Autodesk Inventor part; units mm, degrees
ref_plane "YZ Plane" through (0, 0, 0) normal (1, 0, 0) x (0, 1, 0)
ref_plane "XZ Plane" through (0, 0, 0) normal (0, 1, 0) x (-1, 0, 0)
ref_plane "XY Plane" through (0, 0, 0) normal (0, 0, 1) x (1, 0, 0)
sketch "スケッチ1" plane through (0, 0, 0) normal (0, 1, 0) x (-1, 0, 0)
  line L0 (-6, -5) -> (6, -5)
  line L1 (6, -5) -> (6, 5)
  line L2 (6, 5) -> (-6, 5)
  line L3 (-6, 5) -> (-6, -5)
  line L4 (-6, -5) -> (6, 5) construction
  line L5 (6, -5) -> (-6, 5) construction
  point P0 (0, 0)
  dimension "d0" = 12
  dimension "d1" = 10
extrude "押し出し1" add sketch "スケッチ1" along normal blind 10
sketch "スケッチ3" plane through (0, 10, 0) normal (0, 1, 0) x (1, 0, 0)
  line L0 (6, -5) -> (6, 5)
  line L1 (-6, 5) -> (-6, -5)
  point P0 (0, 0)
  point P1 (3, 0)
  point P2 (-3, 0)
  point P3 (-6, 0)
  dimension "d4" = 3
  dimension "d12" = 3
hole "穴1" at (3, 10, 0) at (-3, 10, 0) direction (0, -1, 0) diameter 3 end through all
sketch "スケッチ4" plane through (6, 0, -5) normal (0, 0, -1) x (-1, 0, 0)
  line L0 (0, 0) -> (12, 0)
  line L1 (12, 0) -> (12, 10)
  point P0 (6, 0)
  point P1 (6, 5)
  point P2 (6, 0)
  point P3 (12, 5)
hole "穴2" at (0, 5, -5) direction (0, 0, 1) diameter 3 end through all
sketch "スケッチ5" plane through (6, 0, 5) normal (1, 0, 0) x (0, 0, -1)
  line L0 (1, 1) -> (9, 1)
  line L1 (9, 1) -> (9, 9)
  line L2 (9, 9) -> (1, 9)
  line L3 (1, 9) -> (1, 1)
  line L4 (1, 1) -> (9, 9) construction
  line L5 (9, 1) -> (1, 9) construction
  line L6 (10, 0) -> (10, 10)
  point P0 (5, 0)
  point P1 (5, 5)
  point P2 (5, 5)
  point P3 (5, 5)
  point P4 (10, 5)
  dimension "d20" = 8
  dimension "d21" = 8
extrude "押し出し2" cut sketch "スケッチ5" against normal blind 12
properties part number "sensor_attach" material "アルミニウム 6061"
Design review of the part built by this model. Coordinates are the model's own, in mm. A direction names the side the tool comes from. Give positions to 0.01 mm unless a question says otherwise; leave off trailing zeros. Order: outer loops, then holes, each group sorted by start corner. A loop starts at its lowest first (then second) coordinate and runs counter-clockwise, first axis right, second up. Notation, with made-up numbers: (-20.75, 88) -> (30.25, 88) arc R16 cw to (30.25, 113) -> close; hole circle Ø6 at (-7.75, 87.25). An arc over 180 degrees is marked (long way). Write each question's results on one line, items separated by ' | '. Start each with the question number.
Q1. Add section A-A on z = -2. Give the boundary of the cut face in (x, y).
Q2. Wall thickness on L1, parallel to Z at x = -3, y = 0.35; L2, parallel to Y at x = -1.75, z = 3; L3, parallel to Z at x = -4.25, y = 2: over which ranges is each line inside the solid? List them lowest first. Write a range as from..to.
Q3. For pin 1 (2.5 mm diameter, centred on x = -3, z = 0, fed in from -Y); pin 2 (5 mm diameter, centred on x = 3, z = -3, fed in from -Y), all flat-tipped, find the tip position at first contact; note any pin that passes through.
Q4. Mouldability with a two-part tool opening along Y and no side actions: class faces 3 (the flat face through (1.2, 3.8, 5)), 4 (the flat face through (0, 0, 0)), 5 (the flat face through (1.4, 4.1, -4)) as +Y half, -Y half, draft (parallel to the pull), parting line (faces both ways), or undercut.
Q5. Add section B-B on z = 0. Give the boundary of the cut face in (x, y), and give its area (3 significant figures).
Q6. Add section C-C on y = 5. Give the boundary of the cut face in (x, z).
Q7. Add section D-D on x = 5.25. Give the boundary of the cut face in (y, z), and give its area (3 significant figures).
Q8. Machinability: for faces 1 (the flat face through (-6, 9.4, -0.1)), 2 (the flat face through (0, 1, 0)), which of the approach directions +Z, -Z, +X, -X, +Y, -Y give a long, thin tool a straight path to every point of the face, cutting with its end or side? Answer none if there is none.
Found:
1) outline: (-6, 0) -> (6, 0) -> (6, 1) -> (-6, 1) -> close; (-6, 9) -> (6, 9) -> (6, 10) -> (-6, 10) -> close
2) L1: z = -5..-1.5, 1.5..5 | L2: y = 0..1, 9..10 | L3: z = -5..-4, 4..5
3) pin 1: passes through | pin 2: stops at y = 0
4) face 3: draft | face 4: -Y half | face 5: undercut
5) outline: (-6, 0) -> (-4.5, 0) -> (-4.5, 1) -> (-6, 1) -> close; (-6, 9) -> (-4.5, 9) -> (-4.5, 10) -> (-6, 10) -> close; (-1.5, 0) -> (1.5, 0) -> (1.5, 1) -> (-1.5, 1) -> close; (-1.5, 9) -> (1.5, 9) -> (1.5, 10) -> (-1.5, 10) -> close; (4.5, 0) -> (6, 0) -> (6, 1) -> (4.5, 1) -> close; (4.5, 9) -> (6, 9) -> (6, 10) -> (4.5, 10) -> close | area: 12.0 mm2
6) outline: (-6, -5) -> (-1.5, -5) -> (-1.5, -4) -> (-6, -4) -> close; (-6, 4) -> (-1.5, 4) -> (-1.5, 5) -> (-6, 5) -> close; (1.5, -5) -> (6, -5) -> (6, -4) -> (1.5, -4) -> close; (1.5, 4) -> (6, 4) -> (6, 5) -> (1.5, 5) -> close
7) outline: (0, -5) -> (10, -5) -> (10, 5) -> (0, 5) -> close; hole (1, -4) -> (9, -4) -> (9, 4) -> (1, 4) -> close | area: 36.0 mm2
8) face 1: +Z, -Z, -X, +Y, -Y | face 2: +X, -X
